from build123d import *

# Parameters (mm, degrees)
F1_DEPTH = 25.4
F3_DEPTH = 25.4


with BuildPart() as f1:
    # F0 (on Front) → F1 (new body)
    with BuildSketch(Plane.XZ):
        Polygon((0, 76.2), (0, 0), (114.3, 0), (114.3, 38.1), (88.9, 76.2), align=None)
    extrude(amount=F1_DEPTH)

    # F2 (on face) → F3 (join)
    with BuildSketch(Plane.XZ.offset(25.4)):
        Polygon((27.145131, 76.2), (1.745131, 76.2), (0, 76.2), (0, 0), (76.2, 0), align=None)
    extrude(amount=F3_DEPTH)


solid = f1.part
Can you work these out from the model? Positions are in its coordinate system, mm. A direction names the side the tool comes from. Give positions to 0.01 mm unless a question says otherwise; leave off trailing zeros. Loops run counter-clockwise (first coordinate to the right, second up) from the corner with the lowest first, then second, coordinate; pieces in that order, holes last. Notation, with made-up numbers: (46.5, 81.5) - (71.5, 81.5) arc R18 ccw to (71.5, 92.5) - close; hole circle Ø11 at (-20.5, 34.25). An arc over 180 degrees is marked (long way). One line per item, written item: value.
(1) On a 3-axis mill with a long thin cutter (end or side, diameter ignored), from which of +Z, -Z, +X, -X, +Y, -Y can I reach the whole of each face in a straight line? I mean faces 1 (the face through (29, -50.8, 30)), 2 (the face through (80, -25.4, 39)). Say none if no direction works.
Verdict:
face 1: +Z, -Z, +X, -X, -Y
face 2: +Z, +X, -Y
(2) If we section it at A-A, the plane y = -11: List the corners of the cut face in (x, z) for me, plus the area to 3 significant figures.
Verdict:
outline: (0, 0) - (114.3, 0) - (114.3, 38.1) - (88.9, 76.2) - (0, 76.2) - close
area: 8,230 mm^2
(3) If we section it at D-D, the plane x = 97: List the corners of the cut face in (y, z) for me, plus the area to 3 significant figures.
Verdict:
outline: (-25.4, 0) - (0, 0) - (0, 64.05) - (-25.4, 64.05) - close
area: 1,630 mm^2
(4) I'm going to push flat-ended pins straight in: pin 1 (5 mm diameter, centred on y = -42.5, z = 44.5, fed in from +X); pin 2 (4 mm diameter, centred on x = 64.5, z = 32, fed in from -Y); pin 3 (6 mm diameter, centred on y = -16.5, z = 55.5, fed in from +X). Where does each tip first touch, or does it pass through?
Verdict:
pin 1: x = 49.16
pin 2: y = -25.4
pin 3: x = 104.7
(5) I need wall thicknesses on line 1 along Y through (x, z) = (79, 64); line 2 along X through (y, z) = (-29.5, 12); line 3 along X through (y, z) = (-25.5, 37). Which ranges of each line are inside material? Lowest first, please.
Verdict:
line 1: -25.4 to 0
line 2: 0 to 68.47
line 3: 0 to 52.38
(6) If we section it at C-C, the plane z = 25.5: List the corners of the cut face in (x, y) for me.
Verdict:
outline: (0, -50.8) - (59.78, -50.8) - (59.78, -25.4) - (114.3, -25.4) - (114.3, 0) - (0, 0) - close
(7) If we section it at B-B, the plane x = 53.5: List the corners of the cut face in (y, z) for me.
Verdict:
outline: (-50.8, 0) - (0, 0) - (0, 76.2) - (-25.4, 76.2) - (-25.4, 35.26) - (-50.8, 35.26) - close
